from build123d import *

# Parameters (mm, degrees)
FILLET_1_R               = 1
SKETCH_3_R               = 7
CUT_EXTRUDE_1_DEPTH      = 10
SKETCH_5_R               = 1.25
CUT_EXTRUDE_2_DEPTH      = 24
SKETCH_6_R               = 1.505
CUT_EXTRUDE_3_DEPTH      = 10
PATTERN_CIRCULAR_1_COUNT = 6


with BuildPart() as part:
    # 草图2 → 旋转1 (revolve)
    with BuildSketch(Plane(origin=(0, 0, 0), x_dir=(0, 0, -1), z_dir=(1, 0, 0))):
        Polygon((20.5, 12), (20.5, 10), (18.086942826, 10), (16.5, 1), (20.5, 1), (20.5, -1), (16.5, -1), (18.086942826, -10), (20.5, -10), (20.5, -12), (15.393316952, -12), (13.630047145, -2), (0, -2), (0, 2), (13.630047145, 2), (15.393316952, 12), align=None)
    revolve(axis=Axis((0, -2, 0), (0, 1, 0)))

    # 圆角1
    fillet_1_edges = [part.edges().sort_by_distance(p)[0] for p in [
        (0, -10, 18.086942826),
        (0, -1, 16.5),
        (0, 1, 16.5),
        (0, 10, 18.086942826),
    ]]
    fillet(fillet_1_edges, radius=FILLET_1_R)

    # 草图3 → 切除-拉伸1 (cut)
    with BuildSketch(Plane(origin=(0, 2, 0), x_dir=(1, 0, 0), z_dir=(0, 1, 0))):
        with Locations(Location((0, 0, 0), (0, 0, 270))):
            Circle(SKETCH_3_R)
    extrude(amount=-CUT_EXTRUDE_1_DEPTH, mode=Mode.SUBTRACT)

    # 草图5 → 切除-拉伸2 (cut)
    with BuildSketch(Plane.XY):
        with Locations(Location((0, 7.923648178, 0), (0, 0, 90.000000002))):
            Circle(SKETCH_5_R)
    cut_extrude_2 = extrude(amount=-CUT_EXTRUDE_2_DEPTH, mode=Mode.SUBTRACT)

    # 镜向1: 切除-拉伸2 across plane
    add(cut_extrude_2.mirror(Plane.ZX), mode=Mode.SUBTRACT)

    # 草图6 → 切除-拉伸3 (cut)
    with BuildSketch(Plane.XZ.offset(2)):
        with Locations(Location((0, 9.5, 0), (0, 0, 270))):
            Circle(SKETCH_6_R)
    cut_extrude_3 = extrude(amount=-CUT_EXTRUDE_3_DEPTH, mode=Mode.SUBTRACT)

    # 阵列(圆周)1: 切除-拉伸3 ×6 about axis
    pattern_circular_1_axis = Axis((0, 0, 0), (0, 1, 0))
    for i in range(1, PATTERN_CIRCULAR_1_COUNT):
        add(cut_extrude_3.rotate(pattern_circular_1_axis, i * 360 / PATTERN_CIRCULAR_1_COUNT), mode=Mode.SUBTRACT)


solid = part.part
Design review of the part built by this model. Coordinates are the model's own, in mm. A direction names the side the tool comes from. Round coordinates to 2 decimals unless told otherwise and drop trailing zeros. Loops run counter-clockwise (first coordinate to the right, second up) from the corner with the lowest first, then second, coordinate; pieces in that order, holes last. Notation, with made-up numbers: M 5.5,71 L 32.5,71 A33 ccw 32.5,103 Z; hole C 70,73 d11. An arc over 180 degrees is marked long. Answer as a JSON object with one key per item and string values.
Item 1: The part is to be moulded in two halves that separate along Z. For faces 4 (the cylindrical face through (-0.375, 9.116, -16.173)), 5 (the cylindrical face through (-0.58, -0.03, 8.11)), 6 (the conical face through (6.428, -2.612, -15.504)), say which applies: pulls with the +Z half, pulls with the -Z half, needs draft (parallel to the pull), parting line crosses it, or undercut.
Answer sheet:
{"face 4": "needs draft", "face 5": "undercut", "face 6": "parting line crosses it"}
Item 2: We need section B-B on y = 4.25. Give the boundary of the cut face in (x, z), and give its area (3 significant figures).
Answer sheet:
{"outline": "C 0,0 d34.15; hole C 0,0 d28.05", "area": "298 mm^2"}
Item 3: Clearance check with flat-ended pins moving along their axes: P1, Ø3.5, axis at x = 8.23, z = 4.75, coming from the +Y side; P2, Ø1.5, axis at x = 11, z = -10, coming from the +Y side; P3, Ø3.5, axis at x = -8.23, z = 4.75, coming from the -Y side; P4, Ø2.5, axis at x = 8.23, z = -4.75, coming from the -Y side. State where each tip first meets the part, or that it passes through.
Answer sheet:
{"P1": "stops at y = 2", "P2": "stops at y = 12", "P3": "stops at y = -2", "P4": "passes through"}
Item 4: We need section A-A on z = -5. State how many separate pieces and enclosed holes the cut face has, and give its area (3 significant figures).
Answer sheet:
{"separate pieces": "4", "enclosed holes": "0", "area": "229 mm^2"}
Item 5: Wall thickness on L1, parallel to Y at x = -15, z = -13; L2, parallel to X at y = 0, z = 0; L3, parallel to Y at x = -8, z = 1: over which ranges is each line inside the solid? List them lowest first. Write a range as from..to.
Answer sheet:
{"L1": "y = -12..-10, -1..1, 10..12", "L2": "x = -20.5..-7, 7..20.5", "L3": "y = -2..2"}
Item 6: Machinability: for faces 1 (the flat face through (6, -1, 17)), 2 (the flat face through (6, -2, -6)), 3 (the flat face through (-15.3, -12, -2.9)), which of the approach directions +Z, -Z, +X, -X, +Y, -Y give a long, thin tool a straight path to every point of the face, cutting with its end or side? Answer none if there is none.
Answer sheet:
{"face 1": "none", "face 2": "-Y", "face 3": "+Z, -Z, +X, -X, -Y"}
